Could you check a few things on this model? Use its own coordinates, in mm. A direction names the side the tool comes from. Coordinates: 2 decimals unless noted, no trailing zeros. Loops run counter-clockwise (first coordinate to the right, second up) from the corner with the lowest first, then second, coordinate; pieces in that order, holes last. Notation, with made-up numbers: M -25.5,38 L 28.5,38 A30 ccw 28.5,72 Z; hole C 42.25,-23 d2. An arc over 180 degrees is marked long. Return JSON: item names as keys, results as strings. Group by question number.
from build123d import *

# Parameters (mm, degrees)
SKETCH1_W           = 230
SKETCH1_H           = 60
BOSS_EXTRUDE1_DEPTH = 3
SKETCH2_W           = 3
SKETCH2_H           = 60
BOSS_EXTRUDE2_DEPTH = 75
CUT_EXTRUDE1_DEPTH  = 75


with BuildPart() as part:
    # Sketch1 → Boss-Extrude1 (new body)
    with BuildSketch(Plane.XY):
        Rectangle(SKETCH1_W, SKETCH1_H)
    extrude(amount=BOSS_EXTRUDE1_DEPTH)

    # Sketch2 → Boss-Extrude2 (add)
    with BuildSketch(Plane(origin=(0, 0, 0), x_dir=(-1, 0, 0), z_dir=(0, 0, -1))):
        Rectangle(SKETCH2_W, SKETCH2_H)
    extrude(amount=BOSS_EXTRUDE2_DEPTH)

    # Sketch3 → Cut-Extrude1 (cut)
    with BuildSketch(Plane(origin=(1.5, 0, 0), x_dir=(0, 0, -1), z_dir=(1, 0, 0))):
        Polygon((75, -10), (0, -30), (75, -30), align=None)
    extrude(amount=-CUT_EXTRUDE1_DEPTH, mode=Mode.SUBTRACT)


solid = part.part
(1) Imagine slicing it at A-A, the plane y = -18. Write out the boundary of the cut face in (x, z).
(2) For faces 1 (the face through (-1.5, 6, -37)), 2 (the face through (57, 0, 0)), 3 (the face through (-2, 0, 3)), which set-ups out of +Z, -Z, +X, -X, +Y, -Y let a thin tool reach every point of the face, with its end or its side?
(3) Imagine slicing it at C-C, the plane x = 52.5. Write out the boundary of the cut face in (y, z), then the cut area to 3 significant figures.
(4) Imagine slicing it at D-D, the plane y = 21.5. Write out the boundary of the cut face in (x, z), then the cut area to 3 significant figures.
(5) Will these pins go through, and if not, where does the flat tip stop? P1, Ø5, axis at y = -12.5, z = -6.5, coming from the -X side; P2, Ø6, axis at y = -12, z = -16.5, coming from the +X side; P3, Ø1, axis at x = 59, y = 10.5, coming from the -Z side.
(6) If I drill on L1, parallel to Z at x = 64, y = 25; L2, parallel to X at y = -7.5, z = -7.5, over which ranges is the centre line in solid material (lowest first)? Write a range as [from, to].
(7) Imagine slicing it at B-B, the plane z = -18. Write out the boundary of the cut face in (x, y).
Checks:
{
 "1": {"outline": "M -115,0 L -1.5,0 L -1.5,-45 L 1.5,-45 L 1.5,0 L 115,0 L 115,3 L -115,3 Z"},
 "2": {"face 1": "-Z, -X, +Y, -Y", "face 2": "-Z, +X, +Y, -Y", "face 3": "+Z, +X, -X, +Y, -Y"},
 "3": {"outline": "M -30,0 L 30,0 L 30,3 L -30,3 Z", "area": "180 mm²"},
 "4": {"outline": "M -115,0 L -1.5,0 L -1.5,-75 L 1.5,-75 L 1.5,0 L 115,0 L 115,3 L -115,3 Z", "area": "915 mm²"},
 "5": {"P1": "x = -1.5", "P2": "x = 1.5", "P3": "z = 0"},
 "6": {"L1": "[0, 3]", "L2": "[-1.5, 1.5]"},
 "7": {"outline": "M -1.5,-25.2 L 1.5,-25.2 L 1.5,30 L -1.5,30 Z"}
}
